Check sheet for the modelled part. Datum: model origin and axes. Units: mm. Face numbers are marked on the shaded views. A direction names the side the tool comes from. Give positions to 0.01 mm unless a question says otherwise; leave off trailing zeros. Loops run counter-clockwise (first coordinate to the right, second up) from the corner with the lowest first, then second, coordinate; pieces in that order, holes last. Notation, with made-up numbers: (-14.5, 79.5) - (22.5, 79.5) arc R22 cw to (22.5, 90.5) - close; hole circle Ø11 at (-4, 44). An arc over 180 degrees is marked (long way). Use one line per item in the form item = value.
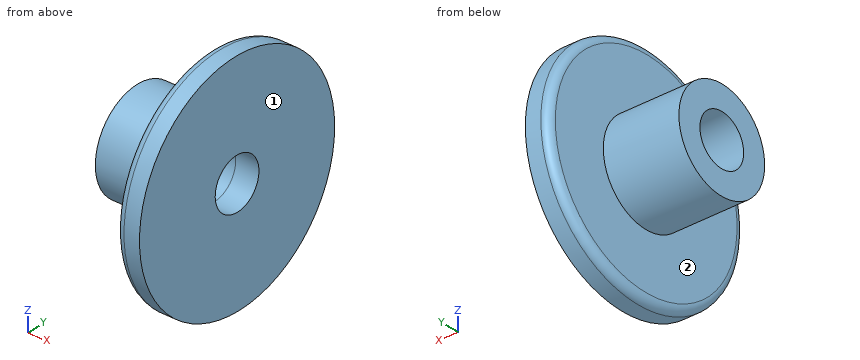
Autodesk Inventor part; units mm, degrees
ref_plane "YZ Plane" through (0, 0, 0) normal (1, 0, 0) x (0, 1, 0)
ref_plane "XZ Plane" through (0, 0, 0) normal (0, 1, 0) x (-1, 0, 0)
ref_plane "XY Plane" through (0, 0, 0) normal (0, 0, 1) x (1, 0, 0)
sketch "Sketch1" plane through (0, 0, 0) normal (1, 0, 0) x (0, 1, 0)
  circle A0 centre (0, 0) radius 14.5
  dimension "d0" = 29
extrude "Extrusion1" add sketch "Sketch1" along normal blind 3
fillet "Fillet1" radius 1 1 edges at (0, -14.5, 0)
sketch "Sketch2" plane through (0, 0, 0) normal (-1, 0, 0) x (0, 0, 1)
  point P0 (0, 0)
sketch "Sketch3" plane through (3, 0, 0) normal (1, 0, 0) x (0, 0, -1)
  circle A0 centre (0, 0) radius 3.25
  dimension "d4" = 6.5
extrude "Extrusion2" cut sketch "Sketch3" against normal blind 3
sketch "Sketch4" plane through (0, 0, 0) normal (-1, 0, 0) x (0, 0, 1)
  circle A0 centre (0, 0) radius 3.25
  circle A1 centre (0, 0) radius 6.375
  dimension "d7" = 12.75
sketch "Sketch5" plane through (0, 0, 0) normal (-1, 0, 0) x (0, 0, 1)
  point P0 (0, 0)
extrude "Extrusion3" add sketch "Sketch4" along normal blind 9.75
properties part number "thiccBB_hubsSlideIn"
Item 1: Access from +Z, -Z, +X, -X, +Y, -Y to the whole of each face (thin tool, end or side, straight path). Record for the marked faces 1 and 2.
Answer block:
face_1 = +Z, -Z, +X, +Y, -Y
face_2 = -X
Item 2: Thickness scan on L1, parallel to Y at x = -5, z = 0 (3 decimals); L2, parallel to Z at x = 1.2, y = 0; L3, parallel to X at y = 8, z = 10.25. Record the ranges inside material, lowest first.
Answer block:
L1 = -6.375 to -3.25, 3.25 to 6.375
L2 = -14.5 to -3.25, 3.25 to 14.5
L3 = 0 to 3
Item 3: Section check A-A on z = 0. Record the boundary of the cut face in (x, y) (3 decimals).
Answer block:
outline = (-9.75, -6.375) - (0, -6.375) - (0, -13.5) arc R1 ccw to (1, -14.5) - (3, -14.5) - (3, -3.25) - (-9.75, -3.25) - close; (-9.75, 3.25) - (3, 3.25) - (3, 14.5) - (1, 14.5) arc R1 ccw to (0, 13.5) - (0, 6.375) - (-9.75, 6.375) - close
Item 4: Gauge pin test, flat ends, axial feed: P1, Ø7.5, axis at y = 0, z = 0, coming from the +X side; P2, Ø3, axis at x = -8, y = -3, coming from the +Z side; P3, Ø3, axis at x = -5, y = -0.5, coming from the -Z side (3 decimals); P4, Ø4, axis at x = 0.5, z = 9, coming from the -Y side. Record the tip position at first contact, or that the pin passes through.
Answer block:
P1 = 3
P2 = 6.2
P3 = -6.375
P4 = -12.67
Item 5: Section check C-C on x = -4.5. Record the boundary of the cut face in (y, z) (3 decimals), then the cut area to 3 significant figures.
Answer block:
outline = circle Ø12.75 at (0, 0); hole circle Ø6.5 at (0, 0)
area = 94.5 mm2
